Check sheet for the modelled part. Datum: model origin and axes. Units: mm. Face numbers are marked on the shaded views. A direction names the side the tool comes from. Round coordinates to 2 decimals unless told otherwise and drop trailing zeros. Loops run counter-clockwise (first coordinate to the right, second up) from the corner with the lowest first, then second, coordinate; pieces in that order, holes last. Notation, with made-up numbers: (-24, 11.25) - (33, 11.25) arc R9 cw to (33, 22.25) - close; hole circle Ø4 at (39.25, 36). An arc over 180 degrees is marked (long way). Put each result on its own line as item: value.
```python
from build123d import *

# Parameters (mm, degrees)
F1_DEPTH = 40
F3_D     = 3
F4_W     = 6
F4_H     = 14
F5_DEPTH = 25


with BuildPart() as f1:
    # F0 (on Front) → F1 (new body)
    with BuildSketch(Plane.XZ):
        Polygon((0, 5), (0, 0), (10, 0), (10, 12), (6, 12), (6, 5), align=None)
    extrude(amount=F1_DEPTH)

    # F3 (through all)
    with Locations(Plane(origin=(6, 0, 0), x_dir=(0, -1, 0), z_dir=(-1, 0, 0))):
        with Locations((35.25, 9), (4.75, 9)):
            Hole(F3_D / 2)

    # F4 (on face) → F5 (cut)
    with BuildSketch(Plane(origin=(0, 0, 0), x_dir=(1, 0, 0), z_dir=(0, 0, -1))):
        with Locations((3, 20)):
            Rectangle(F4_W, F4_H)
    extrude(amount=-F5_DEPTH, mode=Mode.SUBTRACT)


solid = f1.part
```
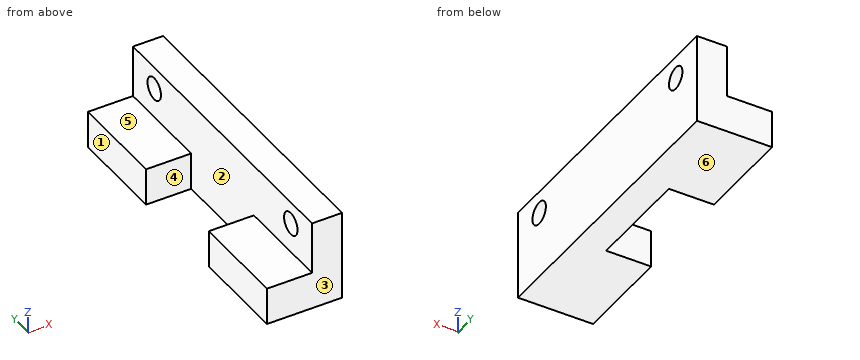
Item 1: Section check A-A on z = 9. Enter the section's corners in (x, y).
Filled sheet:
outline: (6, -40) - (10, -40) - (10, -36.75) - (6, -36.75) - close; (6, -33.75) - (10, -33.75) - (10, -6.25) - (6, -6.25) - close; (6, -3.25) - (10, -3.25) - (10, 0) - (6, 0) - close
Item 2: Go/stop test with flat-tipped pins: pin 1 (3.5 mm diameter, centred on y = -4.75, z = 9, fed in from -X); pin 2 (3 mm diameter, centred on x = 2, y = -36.5, fed in from +Z); pin 3 (2.5 mm diameter, centred on y = -35.25, z = 9, fed in from +X). Record where each tip stops, or that it passes through.
Filled sheet:
pin 1: x = 6
pin 2: z = 5
pin 3: through
Item 3: Release check for a two-part mould opening along Y. For the marked faces 1, 2 and 3 record: +Y half, -Y half, draft (parallel to the pull), parting line (faces both ways), or undercut.
Filled sheet:
face 1: draft
face 2: undercut
face 3: -Y half
Item 4: Section check B-B on x = 1.5. Enter the section's corners in (y, z).
Filled sheet:
outline: (-40, 0) - (-27, 0) - (-27, 5) - (-40, 5) - close; (-13, 0) - (0, 0) - (0, 5) - (-13, 5) - close
Item 5: Tool access check on the marked faces 4, 5 and 6. Record the directions out of +Z, -Z, +X, -X, +Y, -Y that give a thin tool (end or side, any length) a straight path to the whole face; none if there is none.
Filled sheet:
face 4: +Z, -Z, -X
face 5: +Z, -X, +Y, -Y
face 6: -Z, +X, -X, +Y, -Y
Item 6: Thickness scan on line 1 (Z direction, x = 8.95, y = -4.75); line 2 (Y direction, x = 3.5, z = 0.75); line 3 (X direction, y = -33, z = 8.5). Record the ranges inside material, lowest first. Write a range as from..to.
Filled sheet:
line 1: 0..7.5, 10.5..12
line 2: -40..-27, -13..0
line 3: 6..10
Item 7: Section check C-C on y = -35.25. Enter the section's corners in (x, z), then the cut area to 3 significant figures.
Filled sheet:
outline: (0, 0) - (10, 0) - (10, 7.5) - (6, 7.5) - (6, 5) - (0, 5) - close; (6, 10.5) - (10, 10.5) - (10, 12) - (6, 12) - close
area: 66.0 mm²
Item 8: Section check D-D on z = 1. Enter the section's corners in (x, y), then the cut area to 3 significant figures.
Filled sheet:
outline: (0, -40) - (10, -40) - (10, 0) - (0, 0) - (0, -13) - (6, -13) - (6, -27) - (0, -27) - close
area: 316 mm²
